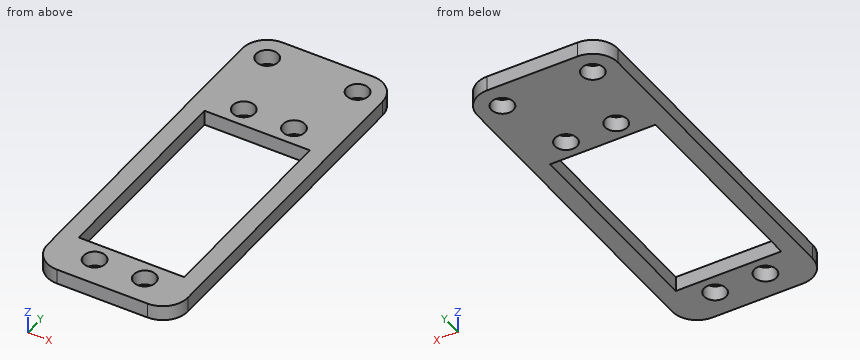
```python
from build123d import *

# Parameters (mm, degrees)
EXTRUDE_1_DEPTH     = 3
SKETCH_3_R          = 2.2
SKETCH_3_W          = 21
SKETCH_3_H          = 41
CUT_EXTRUDE_1_DEPTH = 4
SKETCH_4_R          = 2.2
CUT_EXTRUDE_2_DEPTH = 4


with BuildPart() as part:
    # 草图2 → 凸台-拉伸1 (new body)
    with BuildSketch(Plane.XY):
        with BuildLine():
            Line((-9, -33.5), (9, -33.5))
            ThreePointArc((9, -33.5), (12.535533906, -32.035533906), (14, -28.5))
            Line((14, -28.5), (14, 35))
            ThreePointArc((14, 35), (12.535533906, 38.535533906), (9, 40))
            Line((9, 40), (-9, 40))
            ThreePointArc((-9, 40), (-12.535533906, 38.535533906), (-14, 35))
            Line((-14, 35), (-14, -28.5))
            ThreePointArc((-14, -28.5), (-12.535533906, -32.035533906), (-9, -33.5))
        make_face()
    extrude(amount=EXTRUDE_1_DEPTH)

    # 草图3 → 切除-拉伸1 (cut, through all)
    with BuildSketch(Plane.XY.offset(3)):
        with Locations((-5, 20.815)):
            Circle(SKETCH_3_R)
        with Locations((-5, -27.815)):
            Circle(SKETCH_3_R)
        with Locations((0, -3.5)):
            Rectangle(SKETCH_3_W, SKETCH_3_H)
        with Locations((5, -27.815)):
            Circle(SKETCH_3_R)
        with Locations((5, 20.815)):
            Circle(SKETCH_3_R)
    extrude(amount=-CUT_EXTRUDE_1_DEPTH, mode=Mode.SUBTRACT)

    # 草图4 → 切除-拉伸2 (cut, through all)
    with BuildSketch(Plane.XY.offset(3)):
        with Locations((-9, 35)):
            Circle(SKETCH_4_R)
        with Locations((9, 35)):
            Circle(SKETCH_4_R)
    extrude(amount=-CUT_EXTRUDE_2_DEPTH, mode=Mode.SUBTRACT)


solid = part.part
```
Work out the finished part from the listing and answer in its coordinate system (mm). Round coordinates to 2 decimals unless told otherwise and drop trailing zeros. Write each loop counter-clockwise with the first axis right and the second up, starting at its lowest first coordinate (ties: lowest second). Pieces come first, ordered by that corner, then holes. Notation, with made-up numbers: (49.25, 0.5) - (105.25, 0.5) arc R16 ccw to (105.25, 27.5) - close; hole circle Ø11 at (74, 22.25). An arc over 180 degrees is marked (long way). Return JSON: item names as keys, results as strings. Group by question number.
Q1. Find the intervals of material crossed by L1, parallel to Y at x = 8.75, z = 1.45; L2, parallel to Y at x = 5, z = 1.1 (3 decimals); L3, parallel to X at y = -10.5, z = 0.2, in increasing order.
Q2. This flat-tipped pin is pushed along its axis until it touches: pin 1 Ø7 at (x, y) = (-5, -27.815) entering from +Z. Where does it stop, or does it pass through?
Q3. The part is cut by section C-C on x = -5. Write down the section's boundary in (y, z) (3 decimals).
Q4. The part is cut by section D-D on z = 2.45. Write down the section's boundary in (x, y) (3 decimals), then the cut area to 3 significant figures.
Q5. The part is cut by section B-B on y = 2.5. Write down the section's boundary in (x, z), then the cut area to 3 significant figures.
Q6. The part is cut by section A-A on x = 0. Write down the section's boundary in (y, z).
Solved:
{
 "1": {"L1": "-33.5 to -24, 17 to 32.81, 37.19 to 40", "L2": "-33.5 to -30.015, -25.615 to -24, 17 to 18.615, 23.015 to 40", "L3": "-14 to -10.5, 10.5 to 14"},
 "2": {"pin 1": "z = 3"},
 "3": {"outline": "(-33.5, 0) - (-30.015, 0) - (-30.015, 3) - (-33.5, 3) - close; (-25.615, 0) - (-24, 0) - (-24, 3) - (-25.615, 3) - close; (17, 0) - (18.615, 0) - (18.615, 3) - (17, 3) - close; (23.015, 0) - (40, 0) - (40, 3) - (23.015, 3) - close"},
 "4": {"outline": "(-14, -28.5) arc R5 ccw to (-9, -33.5) - (9, -33.5) arc R5 ccw to (14, -28.5) - (14, 35) arc R5 ccw to (9, 40) - (-9, 40) arc R5 ccw to (-14, 35) - close; hole circle Ø4.4 at (-9, 35); hole (-10.5, -24) - (10.5, -24) - (10.5, 17) - (-10.5, 17) - close; hole circle Ø4.4 at (-5, -27.815); hole circle Ø4.4 at (-5, 20.815); hole circle Ø4.4 at (5, -27.815); hole circle Ø4.4 at (5, 20.815); hole circle Ø4.4 at (9, 35)", "area": "1,080 mm²"},
 "5": {"outline": "(-14, 0) - (-10.5, 0) - (-10.5, 3) - (-14, 3) - close; (10.5, 0) - (14, 0) - (14, 3) - (10.5, 3) - close", "area": "21.0 mm²"},
 "6": {"outline": "(-33.5, 0) - (-24, 0) - (-24, 3) - (-33.5, 3) - close; (17, 0) - (40, 0) - (40, 3) - (17, 3) - close"}
}
